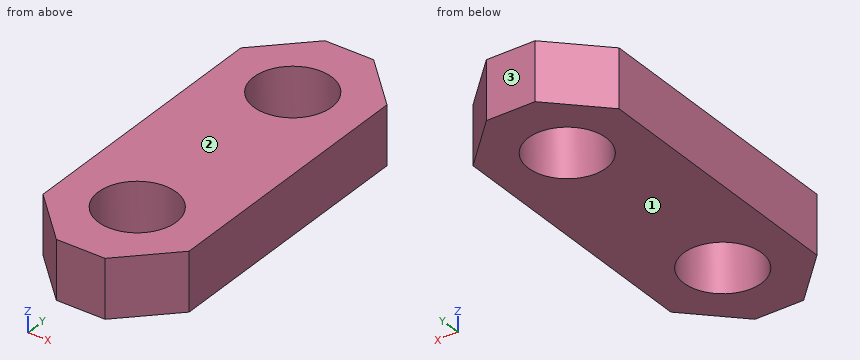
Autodesk Inventor part; units mm, degrees
ref_plane "YZ Plane" through (0, 0, 0) normal (1, 0, 0) x (0, 1, 0)
ref_plane "XZ Plane" through (0, 0, 0) normal (0, 1, 0) x (-1, 0, 0)
ref_plane "XY Plane" through (0, 0, 0) normal (0, 0, 1) x (1, 0, 0)
sketch "Sketch1" plane through (0, 0, 0) normal (0, 0, 1) x (1, 0, 0)
  line L0 (-9, 0) -> (12, 0)
  line L1 (0, 30.4) -> (0, -22.8)
  line L2 (-2.5, 19) -> (2.5, 19)
  line L3 (2.5, 19) -> (7.5, 14)
  line L4 (7.5, 14) -> (7.5, -14)
  line L5 (7.5, -14) -> (2.5, -19)
  line L6 (2.5, -19) -> (-2.5, -19)
  line L7 (-2.5, -19) -> (-7.5, -14)
  line L8 (-7.5, -14) -> (-7.5, 14)
  line L9 (-7.5, 14) -> (-2.5, 19)
  dimension "d0" = 5
  dimension "d1" = 38
  dimension "d2" = 5
  dimension "d3" = 45
  dimension "d5" = 45
  dimension "d6" = 45
  dimension "d7" = 5
  dimension "d8" = 15
  dimension "d10" = 5
extrude "Extrusion1" add sketch "Sketch1" along normal blind 6
sketch "Sketch2" plane through (0, 0, 6) normal (0, 0, 1) x (1, 0, 0)
  line L0 (-2.5, 19) -> (2.5, 19)
  line L1 (2.5, -19) -> (-2.5, -19)
  line L2 (0, 30.4) -> (0, -22.8)
  point P0 (0, 11)
  point P1 (0, -11)
  dimension "d13" = 8
  dimension "d14" = 8
hole "Hole1" at (0, 11, 6) at (0, -11, 6) direction (0, 0, -1) diameter 8 end through all
properties part number "Link"
The listing builds one solid part. Answer for the finished solid, in the listing's coordinates (mm). Face numbers are marked on the shaded views. Give positions to 0.01 mm unless a question says otherwise; leave off trailing zeros. Order: outer loops, then holes, each group sorted by start corner. A loop starts at its lowest first (then second) coordinate and runs counter-clockwise, first axis right, second up. Notation, with made-up numbers: (19, 44.5) -> (60, 44.5) arc R26 ccw to (60, 69.5) -> close; hole circle Ø1 at (29, 5.5). An arc over 180 degrees is marked (long way). Put each result on its own line as item: value.
Item 1: A cutting plane is placed at B-B on x = 0. Give the vertices of the cut face in (y, z).
Established:
outline: (-19, 0) -> (-15, 0) -> (-15, 6) -> (-19, 6) -> close; (-7, 0) -> (7, 0) -> (7, 6) -> (-7, 6) -> close; (15, 0) -> (19, 0) -> (19, 6) -> (15, 6) -> close
Item 2: A cutting plane is placed at D-D on y = -13.5. Give the vertices of the cut face in (x, z).
Established:
outline: (-7.5, 0) -> (-3.12, 0) -> (-3.12, 6) -> (-7.5, 6) -> close; (3.12, 0) -> (7.5, 0) -> (7.5, 6) -> (3.12, 6) -> close
Item 3: For a pull along Z with two mould halves and no side action, classify the marked faces 1, 2 and 3 as released by +Z, released by -Z, zero draft, split by the parting line, or undercut.
Established:
face 1: released by -Z
face 2: released by +Z
face 3: zero draft
Item 4: A cutting plane is placed at A-A on y = 11. Give the vertices of the cut face in (x, z).
Established:
outline: (-7.5, 0) -> (-4, 0) -> (-4, 6) -> (-7.5, 6) -> close; (4, 0) -> (7.5, 0) -> (7.5, 6) -> (4, 6) -> close
Item 5: Given P1, Ø1, axis at x = -5, z = 1, coming from the +Y side; P2, Ø3, axis at x = 1.5, y = 12, coming from the -Z side, each flat-ended and moving along its own axis, determine where each tip first touches the part or whether it passes through.
Established:
P1: stops at y = 17
P2: passes through
Item 6: Straight lines are drawn through the part: line 1 (Y direction, x = 0, z = 2.5); line 2 (X direction, y = 11, z = 2.8); line 3 (Y direction, x = 3.25, z = 4.85). For each, find the intervals that lie inside material, in ascending order.
Established:
line 1: y = -19 to -15, -7 to 7, 15 to 19
line 2: x = -7.5 to -4, 4 to 7.5
line 3: y = -18.25 to -13.33, -8.67 to 8.67, 13.33 to 18.25
Item 7: A cutting plane is placed at C-C on z = 2.75. Give the vertices of the cut face in (x, y).
Established:
outline: (-7.5, -14) -> (-2.5, -19) -> (2.5, -19) -> (7.5, -14) -> (7.5, 14) -> (2.5, 19) -> (-2.5, 19) -> (-7.5, 14) -> close; hole circle Ø8 at (0, -11); hole circle Ø8 at (0, 11)
